CAD build for the part. Positions are in the model's coordinates, mm. A direction names the side the tool comes from. Round coordinates to 2 decimals unless told otherwise and drop trailing zeros. Loops run counter-clockwise (first coordinate to the right, second up) from the corner with the lowest first, then second, coordinate; pieces in that order, holes last. Notation, with made-up numbers: M -36.75,50 L 10.25,50 A24 ccw 10.25,80 Z; hole C 67,48.25 d11. An arc over 180 degrees is marked long. Put each result on its own line as item: value. Start each with the question number.
from build123d import *

# Parameters (mm, degrees)
F1_DEPTH = 25.4
F2_R     = 6.35
F3_DEPTH = 203.2
F4_R     = 6.35
F5_DEPTH = 25.4


with BuildPart() as f1:
    # F0 (on Front) → F1 (new body)
    with BuildSketch(Plane.XZ):
        with BuildLine():
            Line((-254, -12.7), (0, -12.7))
            ThreePointArc((0, -12.7), (12.7, 0), (0, 12.7))
            Line((0, 12.7), (-254, 12.7))
            ThreePointArc((-254, 12.7), (-266.7, 0), (-254, -12.7))
        make_face()
    extrude(amount=F1_DEPTH)

    # F2 (on face) → F3 (join)
    with BuildSketch(Plane.XZ.offset(25.4)):
        with Locations((-254, 0)):
            Circle(F2_R)
        Circle(F2_R)
    extrude(amount=F3_DEPTH)

    # F4 (on face) → F5 (join)
    with BuildSketch(Plane.XZ.offset(228.6)):
        with BuildLine():
            Line((0, 12.7), (-254, 12.7))
            ThreePointArc((-254, 12.7), (-266.7, 0), (-254, -12.7))
            Line((-254, -12.7), (0, -12.7))
            ThreePointArc((0, -12.7), (12.7, 0), (0, 12.7))
        make_face()
        with Locations((-254, 0)):
            Circle(F4_R)
    extrude(amount=F5_DEPTH)


solid = f1.part
(1) Mould opens along Y. For faces 1 (the cylindrical face through (12.697, -241.122, -0.279)), 2 (the cylindrical face through (-247.943, -125.578, 1.907)), 3 (the flat face through (-129, -254, 0)) say: +Y half, -Y half, draft (parallel to the pull), parting line (faces both ways), or undercut.
(2) Flat gauge pins, fed straight in: pin 1 Ø1.5 at (y, z) = (-220, 6.5) entering from -X; pin 2 Ø12 at (y, z) = (-32.5, 2) entering from -X. Where does each tip first touch, or does it go through?
(3) Cut at A-A on x = -77.5. List the corners of the cut face in (y, z), and give its area (3 significant figures).
(4) Cut at B-B on z = 0. List the corners of the cut face in (x, y), and give its area (3 significant figures).
(5) Cut at C-C on y = -211. List the corners of the cut face in (x, z).
(6) Tool access for faces 4 (the cylindrical face through (-266.697, -241.122, 0.279)), 5 (the cylindrical face through (-1.38, -125.58, -6.2)): list every direction of +Z, -Z, +X, -X, +Y, -Y with a clear straight run to the whole face (end or side of a thin tool).
(7) Drill centre lines: line 1 along Y through (x, z) = (-54.5, 10.5); line 2 along X through (y, z) = (-211, -3.25); line 3 along X through (y, z) = (-26, 1.25). Where is each one in solid material? Low to high.
Taken from the geometry:
1. face 1: draft
1. face 2: undercut
1. face 3: -Y half
2. pin 1: x = -256.69
2. pin 2: x = -260.35
3. outline: M -254,-12.7 L -228.6,-12.7 L -228.6,12.7 L -254,12.7 Z; M -25.4,-12.7 L 0,-12.7 L 0,12.7 L -25.4,12.7 Z
3. area: 1,290 mm2
4. outline: M -266.7,-254 L 12.7,-254 L 12.7,-228.6 L 6.35,-228.6 L 6.35,-25.4 L 12.7,-25.4 L 12.7,0 L -266.7,0 L -266.7,-25.4 L -260.35,-25.4 L -260.35,-228.6 L -266.7,-228.6 Z; hole M -247.65,-228.6 L -6.35,-228.6 L -6.35,-25.4 L -247.65,-25.4 Z
4. area: 19,400 mm2
5. outline: C -254,0 d12.7; C 0,0 d12.7
6. face 4: -X, +Y, -Y
6. face 5: none
7. line 1: -254 to -228.6, -25.4 to 0
7. line 2: -259.46 to -248.54, -5.46 to 5.46
7. line 3: -260.23 to -247.77, -6.23 to 6.23
